```python
from build123d import *

# Parameters (mm, degrees)
F0_W     = 6.0909511521
F0_H     = 5
F0_H_2   = 2.6896382868
F0_H_3   = 2.3103617132
F1_DEPTH = 2
F2_DEPTH = 25
F4_R     = 1.99999
F5_R     = 6.305532295
F6_DEPTH = 76


# Not quite as in the source:
# - a fillet or chamfer is up to 0.001 mm smaller than in the source, because OpenCascade refuses the exact size
# - an extrude ends at something that could not be found from the text; its depth is read off the source's solid


with BuildPart() as f1:
    # F0 (on Top) → F1 (new body)
    with BuildSketch(Plane.XY):
        Polygon((-17.4544863403, 13.6900003999), (-20, 13.6900003999), (-20, -18.5), (20, -18.5), (20, 13.6900003999), (17.4544863403, 13.6900003999), (17.4544863403, 11.3796386868), (11.3635351881, 11.3796386868), (11.3635351881, 13.6900003999), (-11.3635351881, 13.6900003999), (-11.3635351881, 11.3796386868), (-17.4544863403, 11.3796386868), align=None)
        with Locations((-14.4090107642, -13.8796386868)):
            Rectangle(F0_W, F0_H, mode=Mode.SUBTRACT)
        with Locations((14.4090107642, -13.8796386868)):
            Rectangle(F0_W, F0_H, mode=Mode.SUBTRACT)
        Polygon((20, 18.5), (-20, 18.5), (-20, 13.6900003999), (-17.4544863403, 13.6900003999), (-17.4544863403, 16.3796386868), (-11.3635351881, 16.3796386868), (-11.3635351881, 13.6900003999), (11.3635351881, 13.6900003999), (11.3635351881, 16.3796386868), (17.4544863403, 16.3796386868), (17.4544863403, 13.6900003999), (20, 13.6900003999), align=None)
        with Locations((14.4090107642, -13.8796386868)):
            Rectangle(F0_W, F0_H)
        with Locations((-14.4090107642, -13.8796386868)):
            Rectangle(F0_W, F0_H)
        with Locations((-14.4090107642, 15.0348195434)):
            Rectangle(F0_W, F0_H_2)
        with Locations((14.4090107642, 15.0348195434)):
            Rectangle(F0_W, F0_H_2)
        with Locations((14.4090107642, 12.5348195434)):
            Rectangle(F0_W, F0_H_3)
        with Locations((-14.4090107642, 12.5348195434)):
            Rectangle(F0_W, F0_H_3)
    extrude(amount=F1_DEPTH)

    # F0 (on Top) → F2 (join)
    with BuildSketch(Plane.XY):
        with Locations((14.4090107642, -13.8796386868)):
            Rectangle(F0_W, F0_H)
        with Locations((14.4090107642, 12.5348195434)):
            Rectangle(F0_W, F0_H_3)
        with Locations((14.4090107642, 15.0348195434)):
            Rectangle(F0_W, F0_H_2)
        with Locations((-14.4090107642, 12.5348195434)):
            Rectangle(F0_W, F0_H_3)
        with Locations((-14.4090107642, 15.0348195434)):
            Rectangle(F0_W, F0_H_2)
        with Locations((-14.4090107642, -13.8796386868)):
            Rectangle(F0_W, F0_H)
    extrude(amount=F2_DEPTH)

    # F4 (radius 2 in the source; OpenCascade refuses exactly that, so slightly less here)
    f4_edges = [f1.edges().sort_by_distance(p)[0] for p in [
        (20, 0, 0),
        (-20, 0, 0),
        (0, -18.5, 0),
    ]]
    fillet(f4_edges, radius=F4_R)

    # F5 (on face) → F6 (cut, through all)
    with BuildSketch(Plane(origin=(0, 13.6900003999, 0), x_dir=(-1, 0, 0), z_dir=(0, 1, 0))):
        with Locations((0, -14.4779002294)):
            Circle(F5_R)
    extrude(amount=F6_DEPTH, mode=Mode.SUBTRACT)


solid = f1.part
```
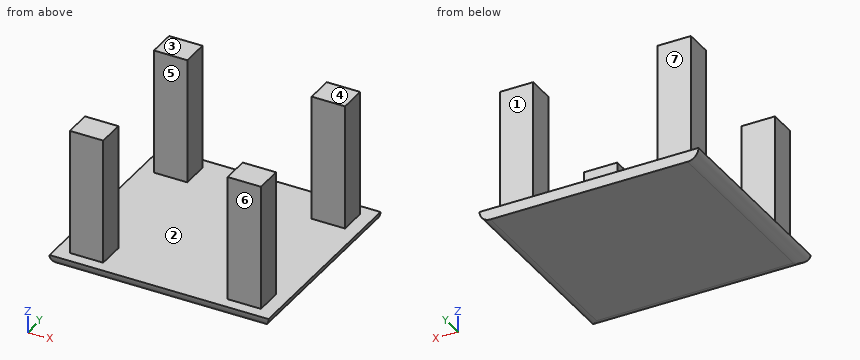
Design review of the part built by this model. Coordinates are the model's own, in mm. Face numbers are marked on the shaded views. A direction names the side the tool comes from. Give positions to 0.01 mm unless a question says otherwise; leave off trailing zeros. Loops run counter-clockwise (first coordinate to the right, second up) from the corner with the lowest first, then second, coordinate; pieces in that order, holes last. Notation, with made-up numbers: (46, 42.25) -> (81, 42.25) arc R15 ccw to (81, 63.25) -> close; hole circle Ø6 at (86, 28.25). An arc over 180 degrees is marked (long way). Write each question's results on one line, items separated by ' | '.
Q1. Wall thickness on L1, parallel to Y at x = -13, z = 22.25; L2, parallel to X at y = -12, z = 16.25; L3, parallel to Z at x = -2, y = -3.5: over which ranges is each line inside the solid? List them lowest first.
Reply:
L1: y = -16.38 to -11.38, 11.38 to 16.38 | L2: x = -17.45 to -11.36, 11.36 to 17.45 | L3: z = 0 to 2
Q2. The part is to be moulded in two halves that separate along Y. For the marked faces 1, 2 and 3, say which applies: +Y half, -Y half, draft (parallel to the pull), parting line (faces both ways), or undercut.
Reply:
face 1: +Y half | face 2: undercut | face 3: draft
Q3. Machinability: for the marked faces 4, 5, 6 and 7, which of the approach directions +Z, -Z, +X, -X, +Y, -Y give a long, thin tool a straight path to every point of the face, cutting with its end or side? Answer none if there is none.
Reply:
face 4: +Z, +X, -X, +Y, -Y | face 5: +Z, +X, -X | face 6: +Z, +X, -X, -Y | face 7: +Z, +X, -X, +Y
Q4. For pin 1 Ø5.5 at (y, z) = (13.5, 13) entering from +X; pin 2 Ø3 at (x, z) = (15.5, 17.5) entering from -Y; pin 3 Ø11 at (x, y) = (-3.5, 9) entering from +Z; pin 4 Ø1 at (x, z) = (-9, 17) entering from +Y, all flat-tipped, find the tip position at first contact; note any pin that passes through.
Reply:
pin 1: stops at x = 17.45 | pin 2: stops at y = -16.38 | pin 3: stops at z = 2 | pin 4: passes through
Q5. Take a section at A-A, the plane z = 7.25. Write out the cut boundary in (x, y).
Reply:
outline: (-17.45, -16.38) -> (-11.36, -16.38) -> (-11.36, -11.38) -> (-17.45, -11.38) -> close; (-17.45, 11.38) -> (-11.36, 11.38) -> (-11.36, 16.38) -> (-17.45, 16.38) -> close; (11.36, -16.38) -> (17.45, -16.38) -> (17.45, -11.38) -> (11.36, -11.38) -> close; (11.36, 11.38) -> (17.45, 11.38) -> (17.45, 16.38) -> (11.36, 16.38) -> close
